Verification items for the finished model (mm, model axes). Coordinates: 2 decimals unless noted, no trailing zeros. Order: outer loops, then holes, each group sorted by start corner. A loop starts at its lowest first (then second) coordinate and runs counter-clockwise, first axis right, second up. Notation, with made-up numbers: (60, -25) -> (66, -25) arc R28 cw to (66, 5) -> close; hole circle Ø4 at (56.25, 30.5). An arc over 180 degrees is marked (long way). Write each question's results on one line, items separated by ' | '. Start each with the question number.
(1) Cross-section at C-C on z = -5. Enter the section's corners in (x, y), and give its area (3 significant figures).
(2) Thickness scan on probe 1 along X at (y, z) = (2.6, -20); probe 2 along Z at (x, y) = (30, 2.5); probe 3 along Z at (x, y) = (4, 1.85). Record the ranges inside material, lowest first. Write a range as [from, to].
(3) Cross-section at D-D on y = 1.3. Give the number of separate pieces and of enclosed holes in the cut face, and give its area (3 significant figures).
(4) Cross-section at B-B on z = 1.5. Enter the section's corners in (x, y).
(5) Cross-section at A-A on x = -10.11. Enter the section's corners in (y, z).
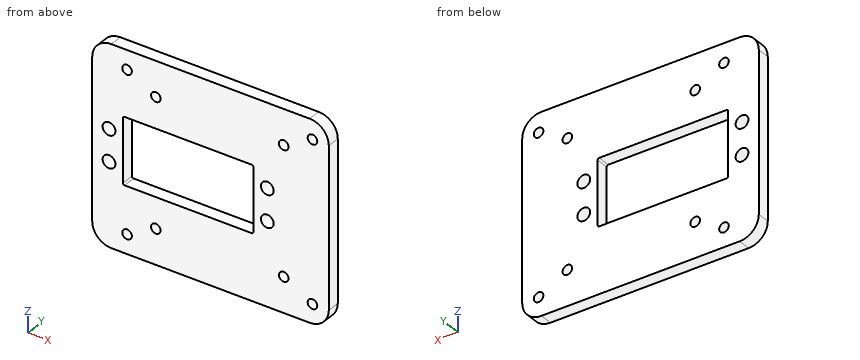
```python
from build123d import *

# Parameters (mm, degrees)
SKETCH_1_W      = 74
SKETCH_1_H      = 62
SKETCH_1_R      = 1.5
SKETCH_1_R_2    = 2
SKETCH_1_W_2    = 40.8
SKETCH_1_H_2    = 20.8
EXTRUDE_1_DEPTH = 4
FILLET_1_R      = 0.5
FILLET_2_R      = 6


with BuildPart() as part:
    # 草图1 → 凸台-拉伸1 (new body)
    with BuildSketch(Plane(origin=(0, 0, 0), x_dir=(1, 0, 0), z_dir=(0, 1, 0))):
        with Locations((7, 0)):
            Rectangle(SKETCH_1_W, SKETCH_1_H)
        with Locations(Location((29.89, 20, 0), (0, 0, 270))):
            Circle(SKETCH_1_R, mode=Mode.SUBTRACT)
        with Locations(Location((29.89, -20, 0), (0, 0, 270))):
            Circle(SKETCH_1_R, mode=Mode.SUBTRACT)
        with Locations(Location((-19.11, -25, 0), (0, 0, 270))):
            Circle(SKETCH_1_R, mode=Mode.SUBTRACT)
        with Locations(Location((-10.11, -20, 0), (0, 0, 270))):
            Circle(SKETCH_1_R, mode=Mode.SUBTRACT)
        with Locations(Location((-24.75, -5, 0), (0, 0, 270))):
            Circle(SKETCH_1_R_2, mode=Mode.SUBTRACT)
        with Locations(Location((24.75, -5, 0), (0, 0, 270))):
            Circle(SKETCH_1_R_2, mode=Mode.SUBTRACT)
        with Locations(Location((-24.75, 5, 0), (0, 0, 270))):
            Circle(SKETCH_1_R_2, mode=Mode.SUBTRACT)
        Rectangle(SKETCH_1_W_2, SKETCH_1_H_2, mode=Mode.SUBTRACT)
        with Locations(Location((-19.11, 25, 0), (0, 0, 270))):
            Circle(SKETCH_1_R, mode=Mode.SUBTRACT)
        with Locations(Location((-10.11, 20, 0), (0, 0, 270))):
            Circle(SKETCH_1_R, mode=Mode.SUBTRACT)
        with Locations(Location((24.75, 5, 0), (0, 0, 270))):
            Circle(SKETCH_1_R_2, mode=Mode.SUBTRACT)
        with Locations(Location((38.89, -25, 0), (0, 0, 270))):
            Circle(SKETCH_1_R, mode=Mode.SUBTRACT)
        with Locations(Location((38.89, 25, 0), (0, 0, 270))):
            Circle(SKETCH_1_R, mode=Mode.SUBTRACT)
    extrude(amount=EXTRUDE_1_DEPTH)

    # 圆角1
    fillet_1_edges = [part.edges().sort_by_distance(p)[0] for p in [
        (20.4, 2, -10.4),
        (-20.4, 2, -10.4),
        (-20.4, 2, 10.4),
        (20.4, 2, 10.4),
    ]]
    fillet(fillet_1_edges, radius=FILLET_1_R)

    # 圆角2
    fillet_2_edges = [part.edges().sort_by_distance(p)[0] for p in [
        (44, 2, 31),
        (-30, 2, 31),
        (-30, 2, -31),
        (44, 2, -31),
    ]]
    fillet(fillet_2_edges, radius=FILLET_2_R)


solid = part.part
```
Results are:
1) outline: (-30, 0) -> (-26.75, 0) -> (-26.75, 4) -> (-30, 4) -> close; (-22.75, 0) -> (-20.4, 0) -> (-20.4, 4) -> (-22.75, 4) -> close; (20.4, 0) -> (22.75, 0) -> (22.75, 4) -> (20.4, 4) -> close; (26.75, 0) -> (44, 0) -> (44, 4) -> (26.75, 4) -> close | area: 101 mm2
2) probe 1: x = [-30, -11.61], [-8.61, 28.39], [31.39, 44] | probe 2: z = [-31, -21.5], [-18.5, 18.5], [21.5, 31] | probe 3: z = [-31, -10.4], [10.4, 31]
3) separate pieces: 1 | enclosed holes: 13 | area: 3,600 mm2
4) outline: (-30, 0) -> (-20.4, 0) -> (-20.4, 4) -> (-30, 4) -> close; (20.4, 0) -> (44, 0) -> (44, 4) -> (20.4, 4) -> close
5) outline: (0, -31) -> (4, -31) -> (4, -21.5) -> (0, -21.5) -> close; (0, -18.5) -> (4, -18.5) -> (4, -10.4) -> (0, -10.4) -> close; (0, 10.4) -> (4, 10.4) -> (4, 18.5) -> (0, 18.5) -> close; (0, 21.5) -> (4, 21.5) -> (4, 31) -> (0, 31) -> close
